```python
from build123d import *

# Parameters (mm, degrees)
EXTRUDE1_DEPTH          = 2.9972
EXTRUDE2_DEPTH          = 5.0038
SKETCH3_R               = 27.75
EXTRUDE3_DEPTH          = 5.5
SKETCH5_R               = 22.25
EXTRUDE4_DEPTH          = 98.06493798
CUT_EXTRUDE1_DEPTH      = 60
CUT_EXTRUDE1_DEPTH_BACK = 60
SKETCH6_W               = 20
SKETCH6_H               = 3
CHAMFER1_SIZE           = 1
SKETCH7_W               = 20
SKETCH7_H               = 8
BOSS_EXTRUDE1_DEPTH     = 15
FILLET1_R               = 2.5
CUT_EXTRUDE2_DEPTH      = 15


with BuildPart() as part:
    # Sketch1 → Extrude1 (new body)
    with BuildSketch(Plane(origin=(0, 0, 0), x_dir=(1, 0, 0), z_dir=(0, 1, 0))):
        with BuildLine():
            Line((-71.882, 54.864), (71.882, 54.864))
            ThreePointArc((71.882, 54.864), (77.539561356, 52.520561356), (79.883, 46.863))
            Line((79.883, 46.863), (79.883, -46.863))
            ThreePointArc((79.883, -46.863), (77.539561356, -52.520561356), (71.882, -54.864))
            Line((71.882, -54.864), (-71.882, -54.864))
            ThreePointArc((-71.882, -54.864), (-77.539561356, -52.520561356), (-79.883, -46.863))
            Line((-79.883, -46.863), (-79.883, 46.863))
            ThreePointArc((-79.883, 46.863), (-77.539561356, 52.520561356), (-71.882, 54.864))
        make_face()
    extrude(amount=EXTRUDE1_DEPTH)

    # Sketch2 → Extrude2 (add)
    with BuildSketch(Plane.XZ):
        with BuildLine():
            Line((68.58, -49.9872), (-68.58, -49.9872))
            ThreePointArc((-68.58, -49.9872), (-73.070128061, -48.127328061), (-74.93, -43.6372))
            Line((-74.93, -43.6372), (-74.93, 43.6372))
            ThreePointArc((-74.93, 43.6372), (-73.070128061, 48.127328061), (-68.58, 49.9872))
            Line((-68.58, 49.9872), (68.58, 49.9872))
            ThreePointArc((68.58, 49.9872), (73.070128061, 48.127328061), (74.93, 43.6372))
            Line((74.93, 43.6372), (74.93, -43.6372))
            ThreePointArc((74.93, -43.6372), (73.070128061, -48.127328061), (68.58, -49.9872))
        make_face()
    extrude(amount=EXTRUDE2_DEPTH)

    # Sketch3 → Extrude3 (cut)
    with BuildSketch(Plane(origin=(0, 2.9972, 0), x_dir=(1, 0, 0), z_dir=(0, 1, 0))):
        with Locations(Location((-15.25, 0, 0), (0, 0, 270))):
            Circle(SKETCH3_R)
    extrude(amount=-EXTRUDE3_DEPTH, mode=Mode.SUBTRACT)

    # Sketch5 → Extrude4 (cut, through all)
    with BuildSketch(Plane(origin=(0, -2.5028, 0), x_dir=(1, 0, 0), z_dir=(0, 1, 0))):
        with Locations(Location((-15.25, 0, 0), (0, 0, 270))):
            Circle(SKETCH5_R)
    extrude(amount=-EXTRUDE4_DEPTH, mode=Mode.SUBTRACT)

    # Sketch6 → Cut-Extrude1 (cut, two sides: drawn at the far end of the back side and taken through both)
    with BuildSketch(Plane.XY.offset(-CUT_EXTRUDE1_DEPTH_BACK)):
        with Locations((30, 1.5)):
            Rectangle(SKETCH6_W, SKETCH6_H)
    extrude(amount=CUT_EXTRUDE1_DEPTH + CUT_EXTRUDE1_DEPTH_BACK, mode=Mode.SUBTRACT)

    # Chamfer1
    chamfer1_edges = [part.edges().sort_by_distance(p)[0] for p in [
        (20, 2.9972, 0),
        (40, 2.9972, 0),
    ]]
    chamfer(chamfer1_edges, length=CHAMFER1_SIZE)

    # Sketch7 → Boss-Extrude1 (add)
    with BuildSketch(Plane(origin=(0, 2.9972, 0), x_dir=(1, 0, 0), z_dir=(0, 1, 0))):
        with Locations((-15.25, -37.5)):
            Rectangle(SKETCH7_W, SKETCH7_H)
    extrude(amount=BOSS_EXTRUDE1_DEPTH)

    # Fillet1
    fillet1_edges = [part.edges().sort_by_distance(p)[0] for p in [
        (-25.25, 10.4972, 33.5),
        (-25.25, 10.4972, 41.5),
        (-5.25, 10.4972, 41.5),
        (-5.25, 10.4972, 33.5),
        (-25.25, 17.9972, 37.5),
        (-15.25, 17.9972, 41.5),
        (-5.25, 17.9972, 37.5),
        (-15.25, 17.9972, 33.5),
    ]]
    fillet(fillet1_edges, radius=FILLET1_R)

    # Sketch8 → Cut-Extrude2 (cut)
    with BuildSketch(Plane(origin=(0, 0, 33.5), x_dir=(-1, 0, 0), z_dir=(0, 0, -1))):
        with BuildLine():
            Line((12.25, 12.5), (18.25, 12.5))
            ThreePointArc((18.25, 12.5), (19.664213562, 11.914213562), (20.25, 10.5))
            Line((20.25, 10.5), (20.25, 9.5))
            ThreePointArc((20.25, 9.5), (19.664213562, 8.085786438), (18.25, 7.5))
            Line((18.25, 7.5), (12.25, 7.5))
            ThreePointArc((12.25, 7.5), (10.835786438, 8.085786438), (10.25, 9.5))
            Line((10.25, 9.5), (10.25, 10.5))
            ThreePointArc((10.25, 10.5), (10.835786438, 11.914213562), (12.25, 12.5))
        make_face()
    extrude(amount=-CUT_EXTRUDE2_DEPTH, mode=Mode.SUBTRACT)


solid = part.part
```
Can you work these out from the model? Positions are in its coordinate system, mm. A direction names the side the tool comes from. Coordinates: 2 decimals unless noted, no trailing zeros. Loops run counter-clockwise (first coordinate to the right, second up) from the corner with the lowest first, then second, coordinate; pieces in that order, holes last.
1) Imagine slicing it at A-A on x = -15.25. List the corners of the cut face in (y, z) for me, plus the area to 3 significant figures.
2) Thinking about a two-plate mould opening in X: for faces 1 (the cylindrical face through (-77.6, 1.48, -52.46)), 2 (the flat face through (76, 0, 0)), 3 (the cylindrical face through (77.6, 1.48, 52.46)), 4 (the cylindrical face through (-0.212, -3.736, -16.399)), which applies, pulls with the +X half, pulls with the -X half, needs draft (parallel to the pull), parting line crosses it, or undercut?
3) Imagine slicing it at D-D on x = 44. List the corners of the cut face in (y, z) for me.
4) For pin 1 (2 mm diameter, centred on x = -54, z = 34.5, fed in from +Y); pin 2 (8 mm diameter, centred on y = 10.5, z = -3.5, fed in from -X); pin 3 (3 mm diameter, centred on x = 39, z = -38.5, fed in from +Y); pin 4 (1.5 mm diameter, centred on x = -32, y = -2, fed in from +Z), each with a flat end and sliding along its axis, tell me the tip position at first contact or that it passes through.
5) Imagine slicing it at B-B on z = 0. List the corners of the cut face in (x, y) for me.
6) Imagine slicing it at C-C on y = 5.25. List the corners of the cut face in (x, z) for me.
7) I need wall thicknesses on probe 1 along X at (y, z) = (1, 0); probe 2 along X at (y, z) = (-0.5, 0); probe 3 along X at (y, z) = (-3.2, 0). Which ranges of each line are inside material? Lowest first, please.
8) Which directions (+Z, -Z, +X, -X, +Y, -Y) give clear straight access to the entire face, cutting with the end or side of a thin tool? Please do faces 5 (the flat face through (-1, -2, 49.987)), 6 (the flat face through (-25.25, 9, 38)), 7 (the cylindrical face through (73.1, -2.5, -48.1)), 8 (the flat face through (-15, 7.5, 37)).
Completed:
1. outline: (-5, -49.99) - (0, -49.99) - (0, -54.86) - (3, -54.86) - (3, -27.75) - (-2.5, -27.75) - (-2.5, -22.25) - (-5, -22.25) - close; (-5, 22.25) - (-2.5, 22.25) - (-2.5, 27.75) - (3, 27.75) - (3, 33.5) - (7.5, 33.5) - (7.5, 41.5) - (3, 41.5) - (3, 54.86) - (0, 54.86) - (0, 49.99) - (-5, 49.99) - close; (12.5, 33.5) - (15.5, 33.5) arc R2.5 ccw to (18, 36) - (18, 39) arc R2.5 ccw to (15.5, 41.5) - (12.5, 41.5) - close
1. area: 490 mm2
2. face 1: pulls with the -X half
2. face 2: needs draft
2. face 3: pulls with the +X half
2. face 4: undercut
3. outline: (-5, -49.99) - (0, -49.99) - (0, -54.86) - (3, -54.86) - (3, 54.86) - (0, 54.86) - (0, 49.99) - (-5, 49.99) - close
4. pin 1: stops at y = 3
4. pin 2: passes through
4. pin 3: stops at y = 2.5
4. pin 4: stops at z = 49.99
5. outline: (-79.88, 0) - (-74.93, 0) - (-74.93, -5) - (-37.5, -5) - (-37.5, -2.5) - (-43, -2.5) - (-43, 3) - (-79.88, 3) - close; (7, -5) - (74.93, -5) - (74.93, 0) - (79.88, 0) - (79.88, 3) - (41, 3) - (40, 2) - (40, 0) - (20, 0) - (20, 2) - (19, 3) - (12.5, 3) - (12.5, -2.5) - (7, -2.5) - close
6. outline: (-25.25, 36) arc R2.5 ccw to (-22.75, 33.5) - (-7.75, 33.5) arc R2.5 ccw to (-5.25, 36) - (-5.25, 39) arc R2.5 ccw to (-7.75, 41.5) - (-22.75, 41.5) arc R2.5 ccw to (-25.25, 39) - close
7. probe 1: x = -79.88 to -43, 12.5 to 20, 40 to 79.88
7. probe 2: x = -74.93 to -43, 12.5 to 74.93
7. probe 3: x = -74.93 to -37.5, 7 to 74.93
8. face 5: +Z, +X, -X, -Y
8. face 6: +Z, -Z, -X, +Y
8. face 7: -Z, +X, -Y
8. face 8: +Z, -Z
